The drawing under review shows one solid part. Ordinate dimensions are in mm from its lowest x, y, z. A direction names the side the tool comes from. Round coordinates to 2 decimals unless told otherwise and drop trailing zeros. Write each loop counter-clockwise with the first axis right and the second up, starting at its lowest first coordinate (ties: lowest second). Pieces come first, ordered by that corner, then holes. Notation, with made-up numbers: M 20,34 L 41,34 A18 ccw 41,67 Z; hole C 4,-11.75 d1. An arc over 180 degrees is marked long. Write item = value, one per line. Start each with the question number.
Item 1: The part is to be moulded in two halves that separate along Y. For the marked faces 3, 4 and 5, say which applies: +Y half, -Y half, draft (parallel to the pull), parting line (faces both ways), or undercut.
Item 2: Take a section at C-C, the plane x = 194. Give the boundary of the cut face in (y, z) (1 decimal).
Item 3: For pin 1 Ø2 at (x, z) = (219, 30.5) entering from +Y; pin 2 Ø5 at (y, z) = (161, 40) entering from +X (1 decimal); pin 3 Ø6 at (y, z) = (114, 13) entering from +X, all flat-tipped, find the tip position at first contact; note any pin that passes through.
Item 4: Take a section at A-A, the plane z = 48.5. Give the boundary of the cut face in (x, y) (1 decimal).
Item 5: Take a section at D-D, the plane z = 22. Give the boundary of the cut face in (x, y) (1 decimal).
Item 6: To check wall thickness, follow line 1 along Y through (x, z) = (223.5, 42) (1 decimal); line 2 along X through (y, z) = (32.5, 12.5); line 3 along Z through (x, y) = (313.5, 78). State the ranges of each line that lie inside material, in increasing order.
Item 7: Tool access review of the marked faces 1 and 2: name each direction out of +Z, -Z, +X, -X, +Y, -Y from which nothing blocks a thin tool from reaching the whole face with its end or side.
Item 8: Take a section at B-B, the plane y = 113. Give the boundary of the cut face in (x, z).
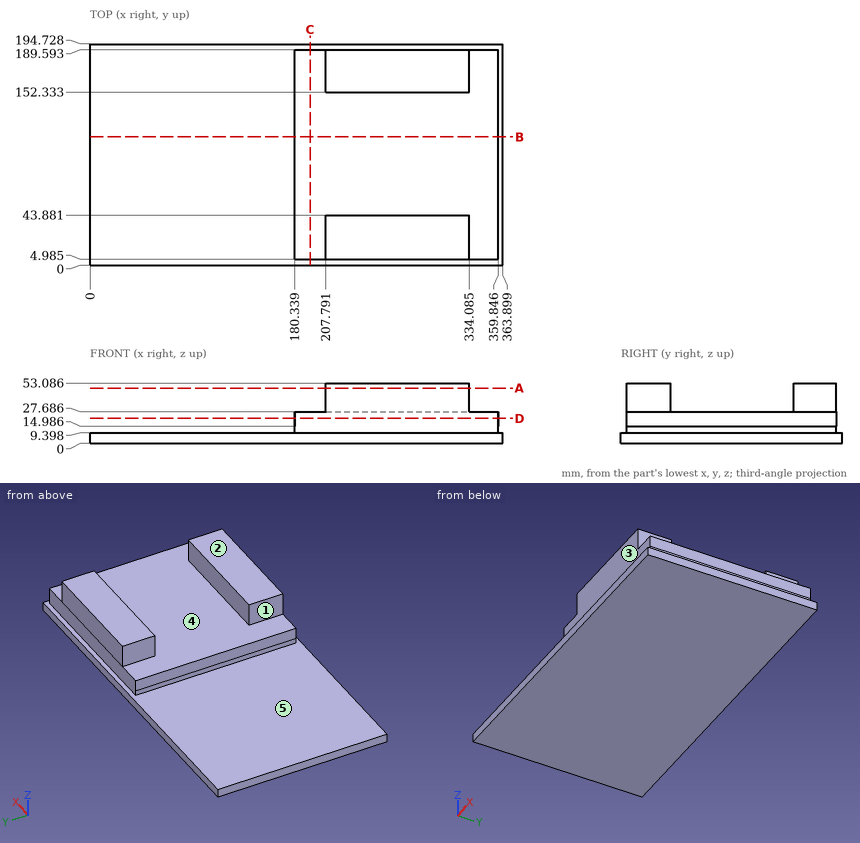
Response values:
q1.face_3 = -Y half
q1.face_4 = undercut
q1.face_5 = draft
q2.outline = M 0,0 L 194.7,0 L 194.7,9.4 L 189.6,9.4 L 189.6,27.7 L 5,27.7 L 5,9.4 L 0,9.4 Z
q3.pin_1 = 189.59
q3.pin_2 = 334.1
q3.pin_3 = 359.85
q4.outline = M 207.8,5 L 334.1,5 L 334.1,43.9 L 207.8,43.9 Z; M 207.8,152.3 L 334.1,152.3 L 334.1,189.6 L 207.8,189.6 Z
q5.outline = M 180.3,5 L 359.8,5 L 359.8,189.6 L 180.3,189.6 Z
q6.line_1 = 5 to 43.9, 152.3 to 189.6
q6.line_2 = 180.34 to 359.85
q6.line_3 = 0 to 27.69
q7.face_1 = +Z, -X, +Y, -Y
q7.face_2 = +Z, +X, -X, +Y, -Y
q8.outline = M 0,0 L 363.9,0 L 363.9,9.4 L 359.85,9.4 L 359.85,27.69 L 180.34,27.69 L 180.34,9.4 L 0,9.4 Z
